Input: part model. Units: mm. Frame: model coordinates. Face numbers are marked on the shaded views. A direction names the side the tool comes from. Round coordinates to 2 decimals unless told otherwise and drop trailing zeros. Order: outer loops, then holes, each group sorted by start corner. A loop starts at its lowest first (then second) coordinate and runs counter-clockwise, first axis right, second up. Notation, with made-up numbers: (-0.75, 60) -> (54.25, 60) arc R11 cw to (54.25, 76) -> close; hole circle Ø6 at (70.5, 11.5). An arc over 180 degrees is marked (long way). Use a Markdown table: item, result.
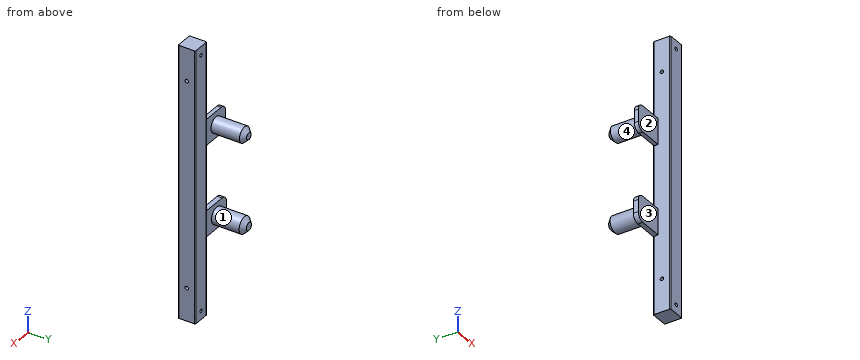
from build123d import *

# Parameters (mm, degrees)
SKETCH_1_W          = 20
SKETCH_1_H          = 20
EXTRUDE_1_DEPTH     = 314
SKETCH_2_R          = 2
CUT_EXTRUDE_1_DEPTH = 314
FILLET_1_R          = 1
SKETCH_3_R          = 2
CUT_EXTRUDE_2_DEPTH = 20
SKETCH_4_W          = 30
SKETCH_4_H          = 5.661352718
SKETCH_4_H_2        = 4.661352718
EXTRUDE_2_DEPTH     = 35
SKETCH_5_R          = 8.993195823
SKETCH_5_R_2        = 9.597903515
EXTRUDE_3_DEPTH     = 38
FILLET_2_R          = 8
CHAMFER_1_SIZE      = 5


with BuildPart() as part:
    # 草图1 → 凸台-拉伸1 (new body)
    with BuildSketch(Plane.XY):
        with Locations((10, 10)):
            Rectangle(SKETCH_1_W, SKETCH_1_H)
    extrude(amount=EXTRUDE_1_DEPTH)

    # 草图2 → 切除-拉伸1 (cut)
    with BuildSketch(Plane(origin=(0, 20, 0), x_dir=(1, 0, 0), z_dir=(0, 1, 0))):
        with Locations(Location((10, -10, 0), (0, 0, 270))):
            Circle(SKETCH_2_R)
        with Locations(Location((10, -304, 0), (0, 0, 270))):
            Circle(SKETCH_2_R)
    extrude(amount=-CUT_EXTRUDE_1_DEPTH, mode=Mode.SUBTRACT)

    # 圆角1
    fillet_1_edges = [part.edges().sort_by_distance(p)[0] for p in [
        (0, 20, 157),
        (20, 20, 157),
        (20, 0, 157),
        (0, 0, 157),
    ]]
    fillet(fillet_1_edges, radius=FILLET_1_R)

    # 草图3 → 切除-拉伸2 (cut)
    with BuildSketch(Plane.ZY):
        with Locations((276, 10)):
            Circle(SKETCH_3_R)
        with Locations((38, 10)):
            Circle(SKETCH_3_R)
    extrude(amount=-CUT_EXTRUDE_2_DEPTH, mode=Mode.SUBTRACT)

    # 草图4 → 凸台-拉伸2 (add)
    with BuildSketch(Plane.ZY):
        with Locations((105, 17.169323641)):
            Rectangle(SKETCH_4_W, SKETCH_4_H)
        with Locations((209, 16.669323641)):
            Rectangle(SKETCH_4_W, SKETCH_4_H_2)
    extrude(amount=EXTRUDE_2_DEPTH)

    # 草图5 → 凸台-拉伸3 (add)
    with BuildSketch(Plane(origin=(0, 19, 0), x_dir=(1, 0, 0), z_dir=(0, 1, 0))):
        with Locations(Location((-17.978292209, -209, 0), (0, 0, 90))):
            Circle(SKETCH_5_R)
        with Locations(Location((-17.978292209, -105, 0), (0, 0, 90))):
            Circle(SKETCH_5_R_2)
    extrude(amount=EXTRUDE_3_DEPTH)

    # 圆角2
    fillet_2_edges = [part.edges().sort_by_distance(p)[0] for p in [
        (-35, 17.169323641, 90),
        (-35, 17.169323641, 120),
        (-35, 16.669323641, 224),
        (-35, 16.669323641, 194),
    ]]
    fillet(fillet_2_edges, radius=FILLET_2_R)

    # 倒角1
    chamfer_1_edges = [part.edges().sort_by_distance(p)[0] for p in [
        (-17.978292209, 57, 217.993195823),
        (-17.978292209, 57, 114.597903515),
    ]]
    chamfer(chamfer_1_edges, length=CHAMFER_1_SIZE)


solid = part.part
1) Set-up query: the marked faces 3 and 4. Return all of +Z, -Z, +X, -X, +Y, -Y with unobstructed straight access to the full face (end or side cutting, diameter ignored); none if empty.
Results found:
| item | result |
|---|---|
| face 3 | +Z, -Z, -X, -Y |
| face 4 | +Y |
2) Cut plane C-C on y = 46. Return loops of the section in (x, z).
Results found:
| item | result |
|---|---|
| outline | circle Ø19.2 at (-17.98, 105); circle Ø17.99 at (-17.98, 209) |
3) Cut plane B-B on z = 209. Return loops of the section in (x, y).
Results found:
| item | result |
|---|---|
| outline | (-35, 14.34) -> (0, 14.34) -> (0, 1) arc R1 ccw to (1, 0) -> (19, 0) arc R1 ccw to (20, 1) -> (20, 19) arc R1 ccw to (19, 20) -> (1, 20) arc R1 ccw to (0, 19) -> (-8.99, 19) -> (-8.99, 52) -> (-13.99, 57) -> (-21.97, 57) -> (-26.97, 52) -> (-26.97, 19) -> (-35, 19) -> close |
4) Pull-direction query (Z, two-part tool) for the marked faces 1 and 2; classes: +Z half, -Z half, draft (parallel to the pull), parting line (faces both ways), or undercut.
Results found:
| item | result |
|---|---|
| face 1 | undercut |
| face 2 | draft |
5) Pin query (flat end, axial travel): pin 1 Ø1.5 at (x, y) = (9.5, 21) entering from -Z; pin 2 Ø1.7 at (x, y) = (-10, 16.5) entering from -Z; pin 3 Ø1.1 at (y, z) = (19.5, 109) entering from +X; pin 4 Ø10 at (x, y) = (-13, 33.5) entering from +Z. Return the tip coordinate at first contact, or that it passes through.
Results found:
| item | result |
|---|---|
| pin 1 | passes through |
| pin 2 | stops at z = 90 |
| pin 3 | stops at x = 20 |
| pin 4 | stops at z = 217.99 |
6) Cut plane A-A on x = -5.5. Return loops of the section in (y, z).
Results found:
| item | result |
|---|---|
| outline | (14.34, 90) -> (20, 90) -> (20, 120) -> (14.34, 120) -> close; (14.34, 194) -> (19, 194) -> (19, 224) -> (14.34, 224) -> close |
7) Line query: L1, parallel to X at y = 14, z = 304; L2, parallel to Z at x = -19, y = 51.5. Output: solid intervals per line, ascending. Write a range as [from, to].
Results found:
| item | result |
|---|---|
| L1 | x = [0, 8], [12, 20] |
| L2 | z = [95.46, 114.54], [200.07, 217.93] |
